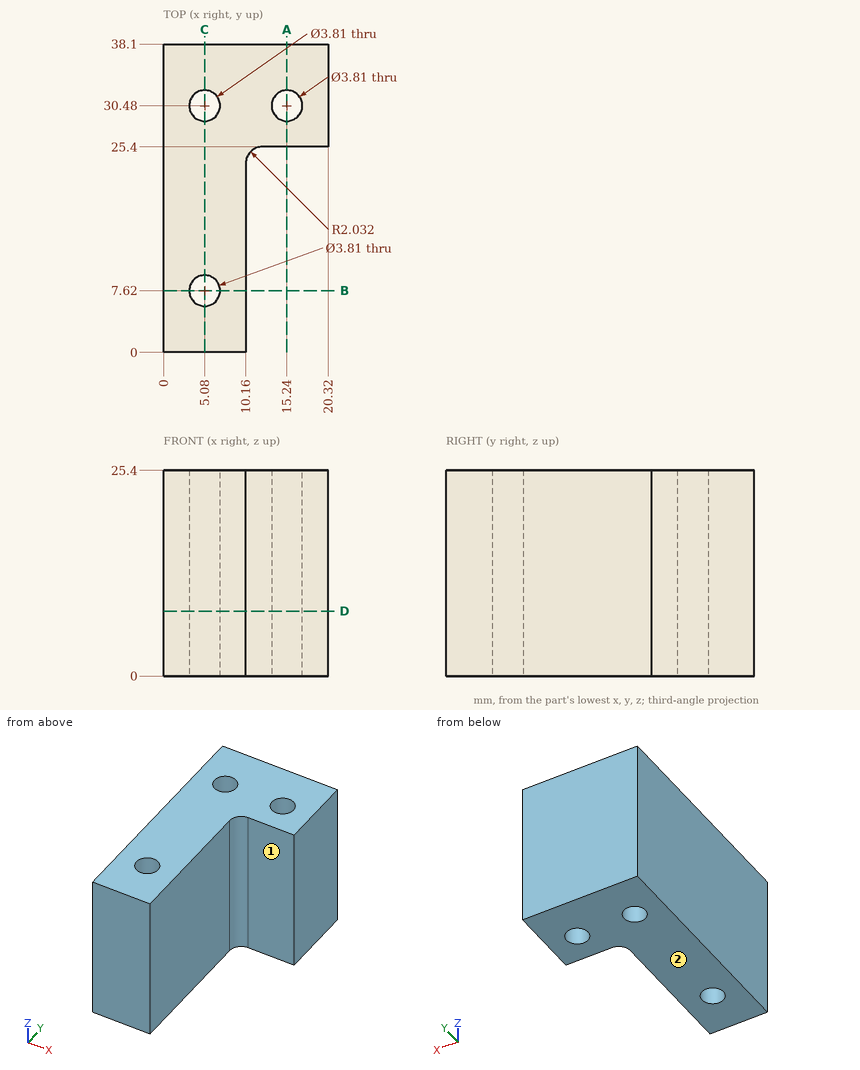
Study the drawing (mm; zero at the part's minimum x, y, z) and answer. A direction names the side the tool comes from. Give positions to 0.01 mm unless a question says otherwise; leave off trailing zeros. Order: outer loops, then holes, each group sorted by start corner. A loop starts at its lowest first (then second) coordinate and runs counter-clockwise, first axis right, second up. Notation, with made-up numbers: (62, 55) -> (119, 55) arc R19 cw to (119, 60) -> close; hole circle Ø6 at (65, -31). An arc over 180 degrees is marked (long way). Write item = value, one per line.
1. A cutting plane is placed at A-A, the plane x = 15.24. Write down the section's boundary in (y, z) (3 decimals).
Numbers:
outline = (25.4, 0) -> (28.575, 0) -> (28.575, 25.4) -> (25.4, 25.4) -> close; (32.385, 0) -> (38.1, 0) -> (38.1, 25.4) -> (32.385, 25.4) -> close
2. A cutting plane is placed at B-B, the plane y = 7.62. Write down the section's boundary in (x, z) (3 decimals), and give its area (3 significant figures).
Numbers:
outline = (0, 0) -> (3.175, 0) -> (3.175, 25.4) -> (0, 25.4) -> close; (6.985, 0) -> (10.16, 0) -> (10.16, 25.4) -> (6.985, 25.4) -> close
area = 161 mm²
3. A cutting plane is placed at C-C, the plane x = 5.08. Write down the section's boundary in (y, z) (3 decimals).
Numbers:
outline = (0, 0) -> (5.715, 0) -> (5.715, 25.4) -> (0, 25.4) -> close; (9.525, 0) -> (28.575, 0) -> (28.575, 25.4) -> (9.525, 25.4) -> close; (32.385, 0) -> (38.1, 0) -> (38.1, 25.4) -> (32.385, 25.4) -> close
4. Straight lines are drawn through the part: line 1 along Y through (x, z) = (5.08, 19) (3 decimals); line 2 along Y through (x, z) = (15, 17.5); line 3 along X through (y, z) = (6, 22). For each, find the intervals that lie inside material, in ascending order.
Numbers:
line_1 = 0 to 5.715, 9.525 to 28.575, 32.385 to 38.1
line_2 = 25.4 to 28.59, 32.37 to 38.1
line_3 = 0 to 4.08, 6.08 to 10.16
5. Given pin 1 (1 mm diameter, centred on y = 19, z = 12, fed in from +X); pin 2 (3 mm diameter, centred on x = 15.24, y = 30.48, fed in from -Z); pin 3 (6.5 mm diameter, centred on x = 14.5, z = 18, fed in from -Y), each flat-ended and moving along its own axis, determine where each tip first touches the part or whether it passes through.
Numbers:
pin_1 = 10.16
pin_2 = through
pin_3 = 25.17
6. For the marked faces 1 and 2, determine the directions among +Z, -Z, +X, -X, +Y, -Y from which every point of the face is accessible in a straight line to the end or side of a thin tool.
Numbers:
face_1 = +Z, -Z, +X, -Y
face_2 = -Z, +X, -X, +Y, -Y
7. A cutting plane is placed at D-D, the plane z = 8. Write down the section's boundary in (x, y) (3 decimals).
Numbers:
outline = (0, 0) -> (10.16, 0) -> (10.16, 23.368) arc R2.032 cw to (12.192, 25.4) -> (20.32, 25.4) -> (20.32, 38.1) -> (0, 38.1) -> close; hole circle Ø3.81 at (5.08, 7.62); hole circle Ø3.81 at (5.08, 30.48); hole circle Ø3.81 at (15.24, 30.48)
